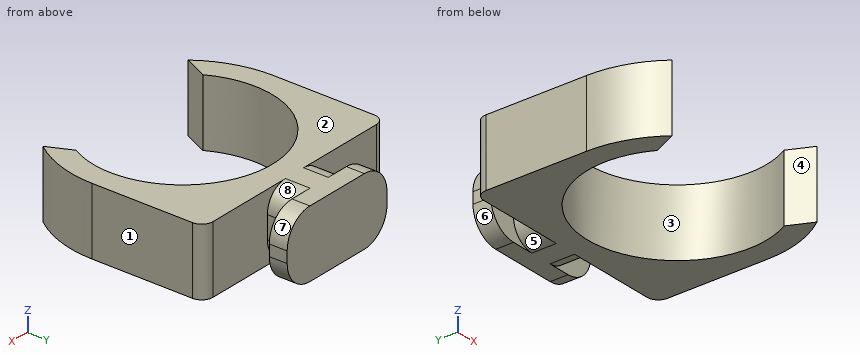
from build123d import *

# Parameters (mm, degrees)
PAD003_DEPTH = 6
FILLET_R     = 2
FILLET001_R  = 2.5
FILLET002_R  = 1


with BuildPart() as part:
    # Sketch023 → Pad003 (new body)
    with BuildSketch(Plane.XY):
        with BuildLine():
            ThreePointArc((7, -3.872983), (0, 8), (-7, -3.872983))
            Line((-7, -3.872983), (-8, -6))
            ThreePointArc((-10, 0), (-9.486833, -3.162278), (-8, -6))
            Line((-10, 0), (-10, 10))
            Line((-10, 10), (-3, 10))
            Line((-3, 10), (-3, 12.2))
            Line((-3, 12.2), (-5.5, 12.2))
            Line((-5.5, 12.2), (-5.5, 13.8))
            Line((-5.5, 13.8), (5.5, 13.8))
            Line((5.5, 13.8), (5.5, 12.2))
            Line((5.5, 12.2), (3, 12.2))
            Line((3, 12.2), (3, 10))
            Line((3, 10), (10, 10))
            Line((10, 0), (10, 10))
            ThreePointArc((8, -6), (9.486833, -3.162278), (10, 0))
            Line((7, -3.872983), (8, -6))
        make_face()
    extrude(amount=PAD003_DEPTH)

    # Fillet
    fillet_edges = [part.edges().sort_by_distance(p)[0] for p in [
        (-3, 11.1, 0),
        (-3, 11.1, 6),
        (3, 11.1, 6),
        (3, 11.1, 0),
    ]]
    fillet(fillet_edges, radius=FILLET_R)

    # Fillet001
    fillet001_edges = [part.edges().sort_by_distance(p)[0] for p in [
        (5.5, 13, 6),
        (5.5, 13, 0),
        (-5.5, 13, 6),
        (-5.5, 13, 0),
    ]]
    fillet(fillet001_edges, radius=FILLET001_R)

    # Fillet002
    fillet002_edges = [part.edges().sort_by_distance(p)[0] for p in [
        (10, 10, 3),
        (-10, 10, 3),
    ]]
    fillet(fillet002_edges, radius=FILLET002_R)


solid = part.part
Input: part model. Units: mm. Frame: model coordinates. Face numbers are marked on the shaded views. A direction names the side the tool comes from. Coordinates: 2 decimals unless noted, no trailing zeros. Loops run counter-clockwise (first coordinate to the right, second up) from the corner with the lowest first, then second, coordinate; pieces in that order, holes last.
(1) Set-up query: the marked faces 4, 5, 6, 7 and 8. Return all of +Z, -Z, +X, -X, +Y, -Y with unobstructed straight access to the full face (end or side cutting, diameter ignored); none if empty.
(2) Section D-D on x = 0. Return the cut outline in (y, z).
(3) First-contact query: pin 1 Ø3 at (x, z) = (6.5, 3) entering from +Y; pin 2 Ø1.1 at (y, z) = (13, 3) entering from +X; pin 3 Ø1.3 at (x, z) = (3.5, 2) entering from -Y; pin 4 Ø0.5 at (y, z) = (13.5, 3) entering from -X. Flat tips, straight axial feed; report the tip coordinate or a pass-through.
(4) Material intervals for probe 1 along X at (y, z) = (12, 3); probe 2 along X at (y, z) = (-3, 2.7); probe 3 along Y at (x, z) = (0, 3.15), sorted ascending.
(5) Pull-direction query (X, two-part tool) for the marked faces 1, 2 and 3; classes: released by +X, released by -X, zero draft, split by the parting line, or undercut.
(6) Section B-B on x = -5.25. Return the cut outline in (y, z), then the cut area to 3 significant figures.
(7) Section A-A on y = 7. Return the cut outline in (x, z).
(8) Section C-C on z = 1.45. Return the cut outline in (x, y), then the cut area to 3 significant figures.
Data:
1. face 4: +Z, -Z, -Y
1. face 5: -Z, -X
1. face 6: -Z, -X, +Y
1. face 7: +Z, +X, +Y
1. face 8: +Z, +X
2. outline: (8, 0) - (13.8, 0) - (13.8, 6) - (8, 6) - close
3. pin 1: stops at y = 13.8
3. pin 2: stops at x = 5.5
3. pin 3: stops at y = 6.84
3. pin 4: stops at x = -5.5
4. probe 1: x = -3 to 3
4. probe 2: x = -9.54 to -7.42, 7.42 to 9.54
4. probe 3: y = 8 to 13.8
5. face 1: released by +X
5. face 2: zero draft
5. face 3: undercut
6. outline: (6.04, 0) - (10, 0) - (10, 6) - (6.04, 6) - close; (12.2, 1.41) - (13.8, 1.41) - (13.8, 4.59) - (12.2, 4.59) - close
6. area: 28.9 mm2
7. outline: (-10, 0) - (-3.87, 0) - (-3.87, 6) - (-10, 6) - close; (3.87, 0) - (10, 0) - (10, 6) - (3.87, 6) - close
8. outline: (-10, 0) arc R10 ccw to (-8, -6) - (-7, -3.87) arc R8 cw (long way) to (7, -3.87) - (8, -6) arc R10 ccw to (10, 0) - (10, 9) arc R1 ccw to (9, 10) - (2.92, 10) - (2.92, 12.2) - (5.27, 12.2) - (5.27, 13.8) - (-5.27, 13.8) - (-5.27, 12.2) - (-2.92, 12.2) - (-2.92, 10) - (-9, 10) arc R1 ccw to (-10, 9) - close
8. area: 150 mm2
